The figure shows three views and two pictorial views of one solid part (mm, origin at its lowest corner). Answer the questions. A direction names the side the tool comes from. Round coordinates to 2 decimals unless told otherwise and drop trailing zeros. Order: outer loops, then holes, each group sorted by start corner. A loop starts at its lowest first (then second) coordinate and runs counter-clockwise, first axis right, second up.
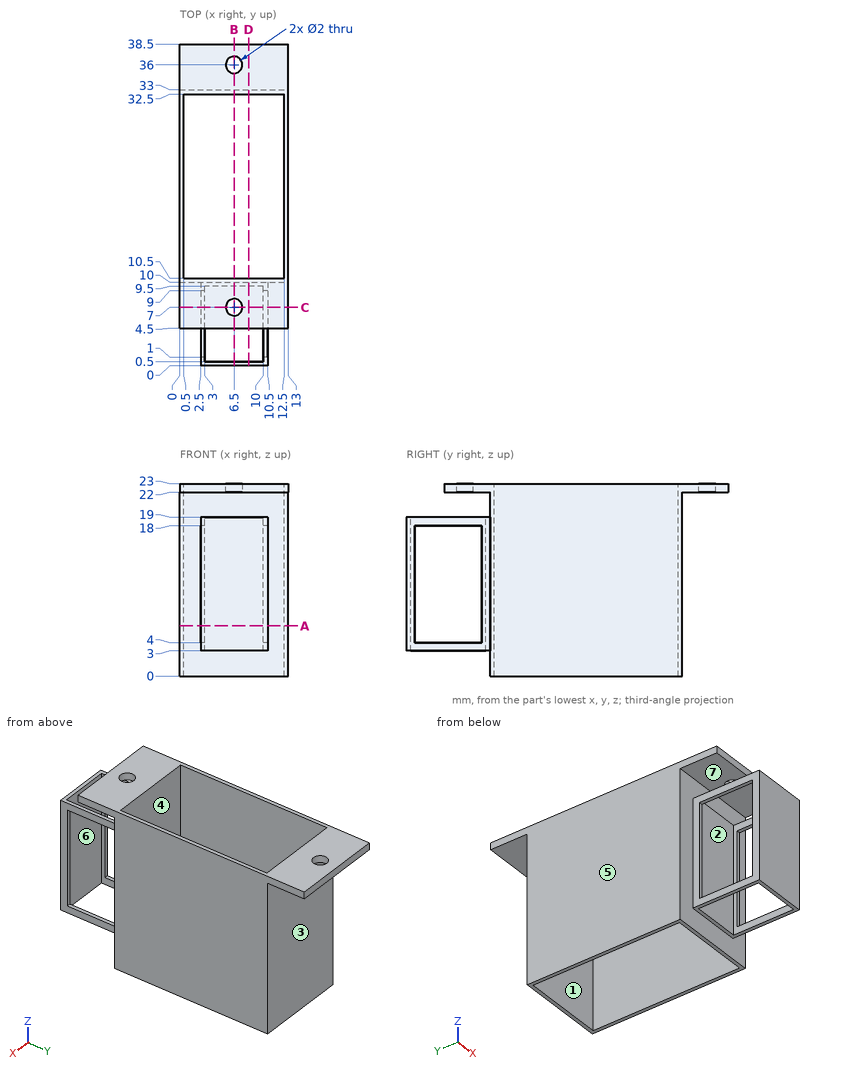
Item 1: Find the intervals of material crossed by line 1 along Y through (x, z) = (6.5, 22.5); line 2 along Y through (x, z) = (6.25, 17); line 3 along X through (y, z) = (36, 22.6), in increasing order.
Item 2: Find section D-D (x = 8.25). Write down the section's boundary in (y, z), plus the area to 3 significant figures.
Item 3: Given pin 1 (8 mm diameter, centred on y = 3, z = 12, fed in from +X); pin 2 (6.5 mm diameter, centred on x = 5, z = 7, fed in from +Y); pin 3 (8 mm diameter, centred on y = 4.5, z = 9.5, fed in from -X), each flat-ended and moving along its own axis, determine where each tip first touches the part or whether it passes through.
Item 4: Find section A-A (z = 6). Write down the section's boundary in (x, y).
Item 5: A tool of negligible diameter and unlimited length cuts with its end or side. For the marked faces 1, 2 and 3, from which of +Z, -Z, +X, -X, +Y, -Y can it reach the whole face along a straight path? Write none if from no direction.
Item 6: Find section C-C (y = 7). Write down the section's boundary in (x, z).
Item 7: Find section B-B (x = 6.5). Write down the section's boundary in (y, z).
Item 8: For a pull along X with two mould halves and no side action, classify the marked faces 4, 5, 6 and 7 as released by +X, released by -X, zero draft, split by the parting line, or undercut.
Model answer:
1. line 1: y = 4.5 to 6, 8 to 10.5, 32.5 to 35, 37 to 38.5
1. line 2: y = 0 to 0.5, 9.5 to 10.5, 32.5 to 33
1. line 3: x = 0 to 5.5, 7.5 to 13
2. outline: (0, 3) - (0.5, 3) - (0.5, 19) - (0, 19) - close; (4.5, 22) - (10, 22) - (10, 19) - (9.5, 19) - (9.5, 3) - (10, 3) - (10, 0) - (10.5, 0) - (10.5, 23) - (4.5, 23) - close; (32.5, 0) - (33, 0) - (33, 22) - (38.5, 22) - (38.5, 23) - (32.5, 23) - close
2. area: 50.0 mm2
3. pin 1: stops at x = 10.5
3. pin 2: stops at y = 33
3. pin 3: stops at x = 2.5
4. outline: (0, 10) - (2.5, 10) - (2.5, 9) - (3, 9) - (3, 9.5) - (10, 9.5) - (10, 9) - (10.5, 9) - (10.5, 10) - (13, 10) - (13, 33) - (0, 33) - close; (2.5, 0) - (10.5, 0) - (10.5, 1) - (10, 1) - (10, 0.5) - (3, 0.5) - (3, 1) - (2.5, 1) - close; hole (0.5, 10.5) - (12.5, 10.5) - (12.5, 32.5) - (0.5, 32.5) - close
5. face 1: +Z, -Z
5. face 2: -Z
5. face 3: -Z, +X, -X, +Y
6. outline: (0, 22) - (5.5, 22) - (5.5, 23) - (0, 23) - close; (2.5, 3) - (3, 3) - (3, 4) - (2.5, 4) - close; (2.5, 18) - (3, 18) - (3, 19) - (2.5, 19) - close; (7.5, 22) - (13, 22) - (13, 23) - (7.5, 23) - close; (10, 3) - (10.5, 3) - (10.5, 4) - (10, 4) - close; (10, 18) - (10.5, 18) - (10.5, 19) - (10, 19) - close
7. outline: (0, 3) - (0.5, 3) - (0.5, 19) - (0, 19) - close; (4.5, 22) - (6, 22) - (6, 23) - (4.5, 23) - close; (8, 22) - (10, 22) - (10, 19) - (9.5, 19) - (9.5, 3) - (10, 3) - (10, 0) - (10.5, 0) - (10.5, 23) - (8, 23) - close; (32.5, 0) - (33, 0) - (33, 22) - (35, 22) - (35, 23) - (32.5, 23) - close; (37, 22) - (38.5, 22) - (38.5, 23) - (37, 23) - close
8. face 4: undercut
8. face 5: released by -X
8. face 6: undercut
8. face 7: zero draft
